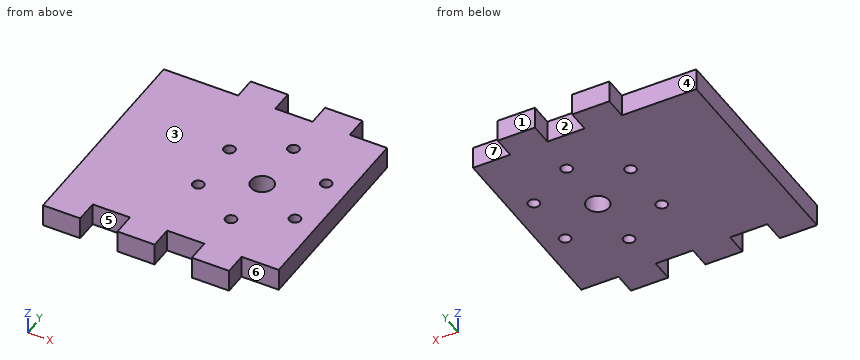
from build123d import *

# Parameters (mm, degrees)
SKETCH1_R           = 0.75
SKETCH1_R_2         = 1.5
BOSS_EXTRUDE1_DEPTH = 3


with BuildPart() as part:
    # Sketch1 → Boss-Extrude1 (new body)
    with BuildSketch(Plane.XY):
        Polygon((10, 0), (10, 3), (15, 3), (15, 0), (20, 0), (20, 3), (25, 3), (25, 0), (30, 0), (30, -26), (25, -26), (25, -29), (20, -29), (20, -26), (15, -26), (15, -29), (10, -29), (10, -26), (5, -26), (5, -29), (0, -29), (0, 0), align=None)
        with Locations((20.5, -5.5)):
            Circle(SKETCH1_R, mode=Mode.SUBTRACT)
        with Locations((26.995190528, -9.25)):
            Circle(SKETCH1_R, mode=Mode.SUBTRACT)
        with Locations((26.995190528, -16.75)):
            Circle(SKETCH1_R, mode=Mode.SUBTRACT)
        with Locations((20.5, -20.5)):
            Circle(SKETCH1_R, mode=Mode.SUBTRACT)
        with Locations((14.004809472, -16.75)):
            Circle(SKETCH1_R, mode=Mode.SUBTRACT)
        with Locations((14.004809472, -9.25)):
            Circle(SKETCH1_R, mode=Mode.SUBTRACT)
        with Locations((20.5, -13)):
            Circle(SKETCH1_R_2, mode=Mode.SUBTRACT)
    extrude(amount=BOSS_EXTRUDE1_DEPTH)


solid = part.part
Check sheet for the modelled part. Datum: model origin and axes. Units: mm. Face numbers are marked on the shaded views. A direction names the side the tool comes from. Round coordinates to 2 decimals unless told otherwise and drop trailing zeros. Loops run counter-clockwise (first coordinate to the right, second up) from the corner with the lowest first, then second, coordinate; pieces in that order, holes last.
1. Set-up check for the marked faces 3, 4, 5, 6 and 7: record each of +Z, -Z, +X, -X, +Y, -Y from which the full face is reachable in a straight line by a thin tool's end or side.
2. Sectioned sample at D-D on y = -16.75. Record the boundary of the cut face in (x, z).
3. Mould release check, pull along X, two halves, no side actions. Record for the marked faces 1 and 2: released by +X, released by -X, zero draft, split by the parting line, or undercut.
4. Scan lines: probe 1 along X at (y, z) = (-27, 0.7); probe 2 along Y at (x, z) = (17, 2); probe 3 along Y at (x, z) = (3.5, 2.1). Record each from-to range of solid material in increasing order.
5. Gauge pin test, flat ends, axial feed: pin 1 Ø1.5 at (x, z) = (6.5, 1) entering from +Y; pin 2 Ø1.5 at (x, z) = (26.5, 1) entering from -Y; pin 3 Ø1.5 at (y, z) = (-27, 1) entering from +X. Record the tip position at first contact, or that the pin passes through.
6. Sectioned sample at A-A on y = -20.5. Record the boundary of the cut face in (x, z), and give its area (3 significant figures).
7. Sectioned sample at C-C on x = 20.5. Record the boundary of the cut face in (y, z), and give its area (3 significant figures).
8. Sectioned sample at B-B on z = 1.5. Give the number of separate pieces and of enclosed holes in the cut face, and give its area (3 significant figures).
Recorded:
1. face 3: +Z, +X, -X, +Y, -Y
1. face 4: +Z, -Z, -X, +Y
1. face 5: +Z, -Z, -Y
1. face 6: +Z, -Z, +X, -Y
1. face 7: +Z, -Z, +X, +Y
2. outline: (0, 0) - (13.25, 0) - (13.25, 3) - (0, 3) - close; (14.75, 0) - (26.25, 0) - (26.25, 3) - (14.75, 3) - close; (27.75, 0) - (30, 0) - (30, 3) - (27.75, 3) - close
3. face 1: zero draft
3. face 2: undercut
4. probe 1: x = 0 to 5, 10 to 15, 20 to 25
4. probe 2: y = -26 to 0
4. probe 3: y = -29 to 0
5. pin 1: stops at y = 0
5. pin 2: stops at y = -26
5. pin 3: stops at x = 25
6. outline: (0, 0) - (19.75, 0) - (19.75, 3) - (0, 3) - close; (21.25, 0) - (30, 0) - (30, 3) - (21.25, 3) - close
6. area: 85.5 mm2
7. outline: (-29, 0) - (-21.25, 0) - (-21.25, 3) - (-29, 3) - close; (-19.75, 0) - (-14.5, 0) - (-14.5, 3) - (-19.75, 3) - close; (-11.5, 0) - (-6.25, 0) - (-6.25, 3) - (-11.5, 3) - close; (-4.75, 0) - (3, 0) - (3, 3) - (-4.75, 3) - close
7. area: 78.0 mm2
8. separate pieces: 1
8. enclosed holes: 7
8. area: 837 mm2
